from build123d import *

# Parameters (mm, degrees)
F1_DEPTH = 25.4


with BuildPart() as f1:
    # F0 (on Top) → F1 (new body)
    with BuildSketch(Plane.XY):
        with BuildLine():
            Line((-63.153848, -8.824982), (-63.153848, -15.414655))
            Line((-63.153848, -15.414655), (-51.874321, -15.414655))
            ThreePointArc((-51.874321, -15.414655), (-47.384193, -13.554783), (-45.524321, -9.064655))
            Line((-45.524321, -9.064655), (-45.524321, 4.344876))
            ThreePointArc((-45.524321, 4.344876), (-43.66445, 8.835004), (-39.174321, 10.694876))
            Line((-39.174321, 10.694876), (25.784801, 10.694876))
            ThreePointArc((25.784801, 10.694876), (30.274929, 8.835004), (32.134801, 4.344876))
            Line((32.134801, 4.344876), (32.134801, -15.414655))
            Line((32.134801, -15.414655), (52.219063, -15.414655))
            Line((52.219063, -15.414655), (52.219063, -8.824982))
            Line((52.219063, -8.824982), (39.631739, -8.824982))
            Line((39.631739, -8.824982), (39.631739, 12.218181))
            ThreePointArc((39.631739, 12.218181), (37.771867, 16.708309), (33.281739, 18.568181))
            Line((33.281739, 18.568181), (-46.313922, 18.568181))
            ThreePointArc((-46.313922, 18.568181), (-50.80405, 16.708309), (-52.663922, 12.218181))
            Line((-52.663922, 12.218181), (-52.663922, -8.824982))
            Line((-52.663922, -8.824982), (-63.153848, -8.824982))
        make_face()
    extrude(amount=F1_DEPTH)


solid = f1.part
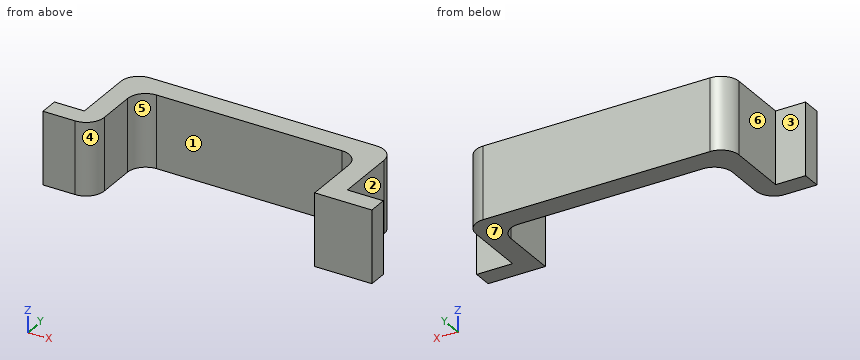
Work out the finished part from the listing and answer in its coordinate system (mm). Face numbers are marked on the shaded views. A direction names the side the tool comes from. Round coordinates to 2 decimals unless told otherwise and drop trailing zeros. Write each loop counter-clockwise with the first axis right and the second up, starting at its lowest first coordinate (ties: lowest second). Pieces come first, ordered by that corner, then holes.
1) The mould has two halves that part along X. Classify the marked faces 4, 5, 6 and 7: pulls with the +X half, pulls with the -X half, needs draft (parallel to the pull), parting line crosses it, or undercut.
2) A cutting plane is placed at D-D (y = 15.5). Give the vertices of the cut face in (x, z), plus the area to 3 significant figures.
3) Given pin 1 Ø10.5 at (y, z) = (4.5, 13) entering from +X; pin 2 Ø3 at (x, z) = (-55.5, 15.5) entering from +Y (3 decimals); pin 3 Ø7.5 at (x, z) = (-8.5, 9) entering from -Y, each flat-ended and moving along its own axis, determine where each tip first touches the part or whether it passes through.
4) A cutting plane is placed at C-C (x = -1.5). Give the vertices of the cut face in (y, z).
5) A cutting plane is placed at B-B (z = 14.75). Give the vertices of the cut face in (x, y).
6) A cutting plane is placed at A-A (y = -2). Give the vertices of the cut face in (x, z), plus the area to 3 significant figures.
7) Straight lines are drawn through the part: line 1 (X direction, y = 2, z = 4.5); line 2 (X direction, y = 12, z = 23); line 3 (Y direction, x = -1, z = 17.75). For each, find the intervals that lie inside material, in ascending order.
8) A tool of negligible diameter and unlimited length cuts with its end or side. For the marked faces 1, 2 and 3, from which of +Z, -Z, +X, -X, +Y, -Y can it reach the whole face along a straight path? Write none if from no direction.
Completed:
1. face 4: undercut
1. face 5: undercut
1. face 6: pulls with the -X half
1. face 7: needs draft
2. outline: (-51.75, 0) - (38.72, 0) - (38.72, 25.4) - (-51.75, 25.4) - close
2. area: 2,300 mm2
3. pin 1: stops at x = 39.63
3. pin 2: stops at y = -8.825
3. pin 3: stops at y = 10.69
4. outline: (10.69, 0) - (18.57, 0) - (18.57, 25.4) - (10.69, 25.4) - close
5. outline: (-63.15, -15.41) - (-51.87, -15.41) arc R6.35 ccw to (-45.52, -9.06) - (-45.52, 4.34) arc R6.35 cw to (-39.17, 10.69) - (25.78, 10.69) arc R6.35 cw to (32.13, 4.34) - (32.13, -15.41) - (52.22, -15.41) - (52.22, -8.82) - (39.63, -8.82) - (39.63, 12.22) arc R6.35 ccw to (33.28, 18.57) - (-46.31, 18.57) arc R6.35 ccw to (-52.66, 12.22) - (-52.66, -8.82) - (-63.15, -8.82) - close
6. outline: (-52.66, 0) - (-45.52, 0) - (-45.52, 25.4) - (-52.66, 25.4) - close; (32.13, 0) - (39.63, 0) - (39.63, 25.4) - (32.13, 25.4) - close
6. area: 372 mm2
7. line 1: x = -52.66 to -45.52, 32.13 to 39.63
7. line 2: x = -52.66 to 39.63
7. line 3: y = 10.69 to 18.57
8. face 1: +Z, -Z, -Y
8. face 2: +Z, -Z, +X, +Y
8. face 3: +Z, -Z, -X, +Y
